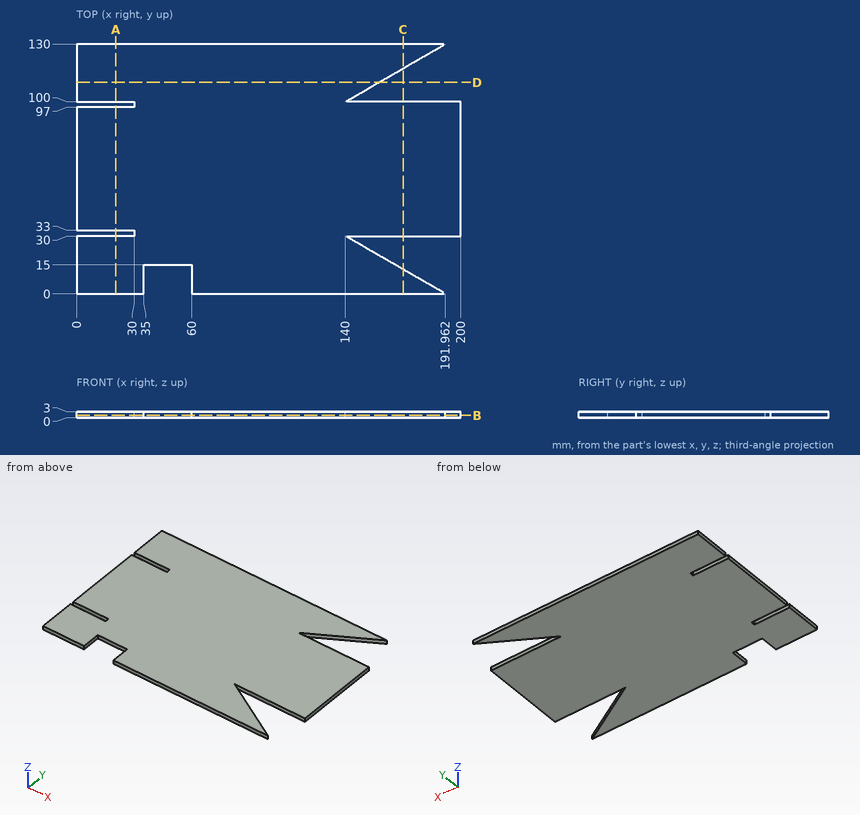
Geometry: see drawing. Coordinates: mm, zero at the bounding-box minimum. Coordinates: 2 decimals unless noted, no trailing zeros. Loops run counter-clockwise (first coordinate to the right, second up) from the corner with the lowest first, then second, coordinate; pieces in that order, holes last. Notation, with made-up numbers: M -38.75,5.5 L 14.25,5.5 A26 cw 14.25,35.5 Z; hole C 62.25,-24.75 d2. An arc over 180 degrees is marked long. Put each result on its own line as item: value. Start each with the question number.
1) Cut plane C-C on x = 170. Return the cut outline in (y, z), then the cut area to 3 significant figures.
2) Ray query, L1, parallel to Y at x = 21.5, z = 0.2; L2, parallel to Y at x = 153, z = 0.6 (1 decimal); L3, parallel to Y at x = 37, z = 2. Return the intervals inside material, ascending. Write a range as from..to.
3) Cut plane D-D on y = 110. Return the cut outline in (x, z), then the cut area to 3 significant figures.
4) Contact query for flat-ended pins moving along their axis: pin 1 Ø0.9 at (x, z) = (50.5, 1) entering from -Y; pin 2 Ø0.9 at (y, z) = (99, 1) entering from -X. Output: stop coordinate, or through.
5) Cut plane A-A on x = 20.5. Return the cut outline in (y, z).
6) Cut plane B-B on z = 1.15. Return the cut outline in (x, y).
The answers:
1. outline: M 0,0 L 12.68,0 L 12.68,3 L 0,3 Z; M 30,0 L 100,0 L 100,3 L 30,3 Z; M 117.32,0 L 130,0 L 130,3 L 117.32,3 Z
1. area: 286 mm²
2. L1: y = 0..30, 33..97, 100..130
2. L2: y = 0..22.5, 30..100, 107.5..130
2. L3: y = 15..130
3. outline: M 0,0 L 157.32,0 L 157.32,3 L 0,3 Z
3. area: 472 mm²
4. pin 1: stops at y = 15
4. pin 2: stops at x = 30
5. outline: M 0,0 L 30,0 L 30,3 L 0,3 Z; M 33,0 L 97,0 L 97,3 L 33,3 Z; M 100,0 L 130,0 L 130,3 L 100,3 Z
6. outline: M 0,0 L 35,0 L 35,15 L 60,15 L 60,0 L 191.96,0 L 140,30 L 200,30 L 200,100 L 140,100 L 191.96,130 L 0,130 L 0,100 L 30,100 L 30,97 L 0,97 L 0,33 L 30,33 L 30,30 L 0,30 Z
